Could you check a few things on this model? Use its own coordinates, in mm. A direction names the side the tool comes from. Coordinates: 2 decimals unless noted, no trailing zeros. Loops run counter-clockwise (first coordinate to the right, second up) from the corner with the lowest first, then second, coordinate; pieces in that order, holes last.
from build123d import *

# Parameters (mm, degrees)
F0_R     = 6.35
F1_DEPTH = 19.05
F2_W     = 25.4
F2_H     = 38.1
F3_DEPTH = 12.7
F4_W     = 7.62
F4_H     = 25.4
F5_DEPTH = 12.7


with BuildPart() as f1:
    # F0 (on Front) → F1 (new body, symmetric)
    with BuildSketch(Plane.XZ):
        with BuildLine():
            ThreePointArc((-12.7, 104.409303), (0, 91.709303), (12.7, 104.409303))
            ThreePointArc((12.7, 104.409303), (0, 117.109303), (-12.7, 104.409303))
        make_face()
        with Locations((0, 104.409303)):
            Circle(F0_R, mode=Mode.SUBTRACT)
        with BuildLine():
            Line((12.7, -22.590697), (12.7, 104.409303))
            ThreePointArc((12.7, 104.409303), (0, 91.709303), (-12.7, 104.409303))
            Line((-12.7, 104.409303), (-12.7, -22.590697))
            ThreePointArc((-12.7, -22.590697), (0, -9.890697), (12.7, -22.590697))
        make_face()
        with BuildLine():
            ThreePointArc((-12.7, -22.590697), (0, -35.290697), (12.7, -22.590697))
            ThreePointArc((12.7, -22.590697), (0, -9.890697), (-12.7, -22.590697))
        make_face()
        with Locations((0, -22.590697)):
            Circle(F0_R, mode=Mode.SUBTRACT)
    extrude(amount=F1_DEPTH, both=True)

    # F2 (on Right) → F3 (cut, symmetric)
    with BuildSketch(Plane.YZ):
        with Locations((0, 103.236585)):
            Rectangle(F2_W, F2_H)
    extrude(amount=F3_DEPTH, both=True, mode=Mode.SUBTRACT)

    # F4 (on Right) → F5 (cut, symmetric)
    with BuildSketch(Plane.YZ):
        with Locations((-16.837219, -23.87516)):
            Rectangle(F4_W, F4_H)
        with Locations((16.182781, -23.87516)):
            Rectangle(F4_W, F4_H)
    extrude(amount=F5_DEPTH, both=True, mode=Mode.SUBTRACT)


solid = f1.part
(1) Imagine slicing it at D-D, the plane y = 16.5. Write out the boundary of the cut face in (x, z), and give its area (3 significant figures).
Answers:
outline: (-12.7, -11.18) - (12.7, -11.18) - (12.7, 104.41) arc R12.7 ccw to (-12.7, 104.41) - close; hole circle Ø12.7 at (0, 104.41)
area: 3,060 mm2
(2) Imagine slicing it at B-B, the plane y = 5.5. Write out the boundary of the cut face in (x, z).
Answers:
outline: (-12.7, -22.59) arc R12.7 ccw to (12.7, -22.59) - (12.7, 84.19) - (-12.7, 84.19) - close; hole circle Ø12.7 at (0, -22.59)
(3) For pin 1 (7 mm diameter, centred on x = 0.5, z = -19.5, fed in from -Y); pin 2 (3.5 mm diameter, centred on x = 0.5, y = 15.5, fed in from -Z); pin 3 (1 mm diameter, centred on x = -2.5, y = -10.5, fed in from +Z), each with a flat end and sliding along its axis, tell me the tip position at first contact or that it passes through.
Answers:
pin 1: stops at y = -13.03
pin 2: stops at z = -11.18
pin 3: stops at z = 84.19
(4) We'd pull the mould along Z, two halves only. Please class faces 6 (the face through (0, 16, -11.175)), 7 (the face through (0, 0, 84.187)), 8 (the face through (-0.827, -15.831, 110.705)), 9 (the face through (0, -19.05, 54)): +Z half, -Z half, draft (parallel to the pull), parting line (faces both ways), or undercut.
Answers:
face 6: -Z half
face 7: +Z half
face 8: undercut
face 9: draft
(5) I need wall thicknesses on probe 1 along Y at (x, z) = (8.5, 88); probe 2 along Z at (x, y) = (0, -15.75); probe 3 along Z at (x, y) = (0, 2.75). Which ranges of each line are inside material? Lowest first, please.
Answers:
probe 1: y = -19.05 to -12.7, 12.7 to 19.05
probe 2: z = -11.18 to 98.06, 110.76 to 117.11
probe 3: z = -35.29 to -28.94, -16.24 to 84.19
(6) Which directions (+Z, -Z, +X, -X, +Y, -Y) give clear straight access to the entire face, cutting with the end or side of a thin tool? Please do faces 1 (the face through (-12.7, 0, 42)), 2 (the face through (0, 12.373, -15)), 3 (the face through (0, 19.05, 54)), 4 (the face through (0, -12.7, 97)), 5 (the face through (0, -13.027, -15)).
Answers:
face 1: +Z, -Z, -X, +Y, -Y
face 2: -Z, +X, -X, +Y
face 3: +Z, -Z, +X, -X, +Y
face 4: +Z, +X, -X
face 5: -Z, +X, -X, -Y
(7) Imagine slicing it at A-A, the plane x = 0. Write out the boundary of the cut face in (y, z), and give its area (3 significant figures).
Answers:
outline: (-19.05, -11.18) - (-13.03, -11.18) - (-13.03, -16.24) - (12.37, -16.24) - (12.37, -11.18) - (19.05, -11.18) - (19.05, 98.06) - (12.7, 98.06) - (12.7, 84.19) - (-12.7, 84.19) - (-12.7, 98.06) - (-19.05, 98.06) - close; (-19.05, 110.76) - (-12.7, 110.76) - (-12.7, 117.11) - (-19.05, 117.11) - close; (-13.03, -35.29) - (12.37, -35.29) - (12.37, -28.94) - (-13.03, -28.94) - close; (12.7, 110.76) - (19.05, 110.76) - (19.05, 117.11) - (12.7, 117.11) - close
area: 4,180 mm2
(8) Imagine slicing it at C-C, the plane x = 7.75. Write out the boundary of the cut face in (y, z), and give its area (3 significant figures).
Answers:
outline: (-19.05, -11.18) - (-13.03, -11.18) - (-13.03, -32.65) - (12.37, -32.65) - (12.37, -11.18) - (19.05, -11.18) - (19.05, 114.47) - (12.7, 114.47) - (12.7, 84.19) - (-12.7, 84.19) - (-12.7, 114.47) - (-19.05, 114.47) - close
area: 4,560 mm2
